from build123d import *

# Parameters (mm, degrees)
F1_DEPTH = 25.4
F3_DEPTH = 25.4


with BuildPart() as f1:
    # F0 (on Front) → F1 (new body)
    with BuildSketch(Plane.XZ):
        Polygon((58.0202316056, 36.9197579437), (40.3588265181, 75.2369578606), (20.0064992297, 37.2961324534), align=None)
        Polygon((40.3588265181, 0), (20.0064992297, 37.2961324534), (0, 0), align=None)
        Polygon((58.0202316056, 36.9197579437), (20.0064992297, 37.2961324534), (40.3588265181, 0), align=None)
        Polygon((75.0375189384, 0), (58.0202316056, 36.9197579437), (40.3588265181, 0), align=None)
    extrude(amount=F1_DEPTH)

    # F2 (on Front) → F3 (cut, symmetric)
    with BuildSketch(Plane.XZ):
        Polygon((56.622825563, 32.7289290726), (19.8782272637, 32.7289290726), (40.0576405227, 7.730553858), align=None)
    extrude(amount=F3_DEPTH, both=True, mode=Mode.SUBTRACT)


solid = f1.part
Read the model definition and answer for the solid it produces. Units are mm, in the model's axes. A direction names the side the tool comes from. Give positions to 0.01 mm unless a question says otherwise; leave off trailing zeros. Write each loop counter-clockwise with the first axis right and the second up, starting at its lowest first coordinate (ties: lowest second). Pieces come first, ordered by that corner, then holes. Notation, with made-up numbers: (5, 82.25) - (32, 82.25) arc R5 cw to (32, 88.25) - close; hole circle Ø2 at (69.25, -34.5). An arc over 180 degrees is marked (long way). Use CSV: the item, a comma, the result in double quotes. Start each with the question number.
Item 1: Flat-ended cylindrical pins translate along their axes: P1, Ø6, axis at y = -17, z = 52.5, coming from the +X side; P2, Ø1, axis at x = 13.5, y = -11, coming from the +Z side; P3, Ø1, axis at y = -5.5, z = 25, coming from the -X side. Find the tip coordinate at first contact, or state that the pin passes through.
Item 2: The part is cut by section A-A, the plane y = -7.75. Give the vertices of the cut face in (x, z).
Item 3: The part is cut by section B-B, the plane x = 51. Give the vertices of the cut face in (y, z), and give its area (3 significant figures).
Item 4: The part is cut by section C-C, the plane z = 21.5. Give the vertices of the cut face in (x, y).
Item 5: The part is cut by section D-D, the plane x = 12.5. Give the vertices of the cut face in (y, z), and give its area (3 significant figures).
Item 6: For faces 5 (the flat face through (29.83, -12.88, 20.4)), 6 (the flat face through (29, 0, 21)), determine the directions among +Z, -Z, +X, -X, +Y, -Y from which every point of the face is accessible in a straight line to the end or side of a thin tool.
Item 7: The mould has two halves that part along X. Classify faces 1 (the flat face through (39, -13, 32.729)), 2 (the flat face through (37, -13, 0)), 3 (the flat face through (48.22, -12.88, 20.05)), 4 (the flat face through (20.462, -12.522, 38.145)): pulls with the +X half, pulls with the -X half, needs draft (parallel to the pull), parting line crosses it, or undercut.
Item 8: Consider line 1 (X direction, y = -18, z = 11); line 2 (Z direction, x = 45.5, y = -2.75); line 3 (Z direction, x = 51.5, y = -16.25). Determine where each line is inside the solid, lowest interval first.
Taken from the geometry:
1,P1,"x = 52.22"
1,P2,"z = 26.1"
1,P3,"x = 13.14"
2,outline,"(0, 0) - (75.04, 0) - (40.36, 75.24) - close; hole (19.88, 32.73) - (40.06, 7.73) - (56.62, 32.73) - close"
3,outline,"(-25.4, 0) - (0, 0) - (0, 24.24) - (-25.4, 24.24) - close; (-25.4, 32.73) - (0, 32.73) - (0, 52.15) - (-25.4, 52.15) - close"
3,area,"1,110 mm2"
4,outline,"(11.53, -25.4) - (28.94, -25.4) - (28.94, 0) - (11.53, 0) - close; (49.18, -25.4) - (65.13, -25.4) - (65.13, 0) - (49.18, 0) - close"
5,outline,"(-25.4, 0) - (0, 0) - (0, 23.3) - (-25.4, 23.3) - close"
5,area,"592 mm2"
6,face 5,"+Y, -Y"
6,face 6,"+Z, -Z, +X, -X, +Y"
7,face 1,"undercut"
7,face 2,"needs draft"
7,face 3,"undercut"
7,face 4,"pulls with the -X half"
8,line 1,"5.9 to 37.42, 42.22 to 69.97"
8,line 2,"0 to 15.94, 32.73 to 64.08"
8,line 3,"0 to 25, 32.73 to 51.07"
